Source: CAD feature listing. Evaluate the final solid. Frame: model axes, mm. A direction names the side the tool comes from. Round coordinates to 2 decimals unless told otherwise and drop trailing zeros. Loops run counter-clockwise (first coordinate to the right, second up) from the corner with the lowest first, then second, coordinate; pieces in that order, holes last. Notation, with made-up numbers: (71.25, 72) -> (87.25, 72) arc R24 ccw to (87.25, 91) -> close; hole circle Ø4 at (-2, -16.5). An arc over 180 degrees is marked (long way). Write item = value, one per line.
from build123d import *

# Parameters (mm, degrees)
SKETCH1_W                 = 33
SKETCH1_H                 = 33
BOSS_EXTRUDE1_DEPTH       = 10
SHELL1_T                  = -4
SHELL1_THICKNESS_2_FACE_W = 2
SHELL1_THICKNESS_2_FACE_H = 29
SHELL1_THICKNESS_2_DEPTH  = 1.5
SHELL1_THICKNESS_3_FACE_W = 29
SHELL1_THICKNESS_3_FACE_H = 2
SHELL1_THICKNESS_3_DEPTH  = 1.5
SKETCH3_R                 = 10
CUT_EXTRUDE1_DEPTH        = 10
SKETCH5_R                 = 4
BOSS_EXTRUDE2_DEPTH       = 30


with BuildPart() as part:
    # Sketch1 → Boss-Extrude1 (new body)
    with BuildSketch(Plane.XY):
        with Locations((4.463597679, 4.532591876)):
            Rectangle(SKETCH1_W, SKETCH1_H)
    extrude(amount=BOSS_EXTRUDE1_DEPTH)

    # Shell1
    shell1_openings = [part.faces().sort_by_distance(p)[0] for p in [
        (4.463597679, -11.967408124, 5),
    ]]
    offset(amount=SHELL1_T, openings=shell1_openings, kind=Kind.INTERSECTION)

    # Shell1 thickness 2 face (on inner face of the shell) → Shell1 thickness 2 (cut)
    with BuildSketch(Plane(origin=(16.963597679, 2.532591876, 5), x_dir=(0, 0, 1), z_dir=(1, 0, 0))):
        Rectangle(SHELL1_THICKNESS_2_FACE_W, SHELL1_THICKNESS_2_FACE_H)
    extrude(amount=SHELL1_THICKNESS_2_DEPTH, mode=Mode.SUBTRACT)

    # Shell1 thickness 3 face (on inner face of the shell) → Shell1 thickness 3 (cut)
    with BuildSketch(Plane(origin=(-8.036402321, 2.532591876, 5), x_dir=(0, -1, 0), z_dir=(-1, 0, 0))):
        Rectangle(SHELL1_THICKNESS_3_FACE_W, SHELL1_THICKNESS_3_FACE_H)
    extrude(amount=SHELL1_THICKNESS_3_DEPTH, mode=Mode.SUBTRACT)

    # Sketch3 → Cut-Extrude1 (cut)
    with BuildSketch(Plane.XY.offset(10)):
        with Locations((4.463597679, 4.532591876)):
            Circle(SKETCH3_R)
    extrude(amount=-CUT_EXTRUDE1_DEPTH, mode=Mode.SUBTRACT)

    # Sketch5 → Boss-Extrude2 (add)
    with BuildSketch(Plane(origin=(0, 21.032591876, 0), x_dir=(1, 0, 0), z_dir=(0, 1, 0))):
        with Locations(Location((4.463597679, -5, 0), (0, 0, 270))):
            Circle(SKETCH5_R)
    extrude(amount=BOSS_EXTRUDE2_DEPTH)


solid = part.part
1. Set-up query: faces 4 (the face through (8.43, 35.82, 4.48)), 5 (the face through (-9.536, 3, 5)), 6 (the face through (2.3, -5.23, 2.03)). Return all of +Z, -Z, +X, -X, +Y, -Y with unobstructed straight access to the full face (end or side cutting, diameter ignored); none if empty.
Evaluation:
face_4 = +Y
face_5 = -Y
face_6 = +Z, -Z
2. Line query: probe 1 along Z at (x, y) = (-9, 17); probe 2 along Y at (x, z) = (5, 6.25); probe 3 along X at (y, z) = (42, 4.75). Output: solid intervals per line, ascending. Write a range as from..to.
Evaluation:
probe_1 = 0..4, 6..10
probe_2 = -11.97..-5.45, 14.52..51.03
probe_3 = 0.47..8.46
3. Section query A-A (x = 17.5). Return the cut outline in (y, z).
Evaluation:
outline = (-11.97, 0) -> (21.03, 0) -> (21.03, 10) -> (-11.97, 10) -> (-11.97, 6) -> (17.03, 6) -> (17.03, 4) -> (-11.97, 4) -> close
4. Contact query for flat-ended pins moving along their axis: pin 1 Ø14 at (x, y) = (3.5, 4.5) entering from -Z; pin 2 Ø4 at (y, z) = (42, 1) entering from -X; pin 3 Ø0.6 at (x, z) = (5, 5) entering from -Y; pin 4 Ø1 at (y, z) = (24, 4) entering from +X. Output: stop coordinate, or through.
Evaluation:
pin_1 = through
pin_2 = 1
pin_3 = 17.03
pin_4 = 8.43
5. Mould query, pull axis Z, two halves, no side actions, for faces 1 (the face through (0.6, 21.033, 2.7)), 2 (the face through (11, -4, 6)), 3 (the face through (-3, 12, 10)). Classes: released by +Z, released by -Z, zero draft, split by the parting line, or undercut.
Evaluation:
face_1 = zero draft
face_2 = undercut
face_3 = released by +Z
6. Section query D-D (x = 11.5). Return the cut outline in (y, z).
Evaluation:
outline = (-11.97, 0) -> (-2.57, 0) -> (-2.57, 4) -> (-11.97, 4) -> close; (-11.97, 6) -> (-2.57, 6) -> (-2.57, 10) -> (-11.97, 10) -> close; (11.64, 0) -> (21.03, 0) -> (21.03, 10) -> (11.64, 10) -> (11.64, 6) -> (17.03, 6) -> (17.03, 4) -> (11.64, 4) -> close
7. Section query C-C (z = 8). Return the cut outline in (x, y), then the cut area to 3 significant figures.
Evaluation:
outline = (-12.04, -11.97) -> (20.96, -11.97) -> (20.96, 21.03) -> (7.11, 21.03) -> (7.11, 51.03) -> (1.82, 51.03) -> (1.82, 21.03) -> (-12.04, 21.03) -> close; hole circle Ø20 at (4.46, 4.53)
area = 934 mm²
8. Section query B-B (z = 5). Return the cut outline in (x, y), then the cut area to 3 significant figures.
Evaluation:
outline = (-12.04, -11.97) -> (-9.54, -11.97) -> (-9.54, 17.03) -> (18.46, 17.03) -> (18.46, -11.97) -> (20.96, -11.97) -> (20.96, 21.03) -> (8.46, 21.03) -> (8.46, 51.03) -> (0.46, 51.03) -> (0.46, 21.03) -> (-12.04, 21.03) -> close
area = 517 mm²
